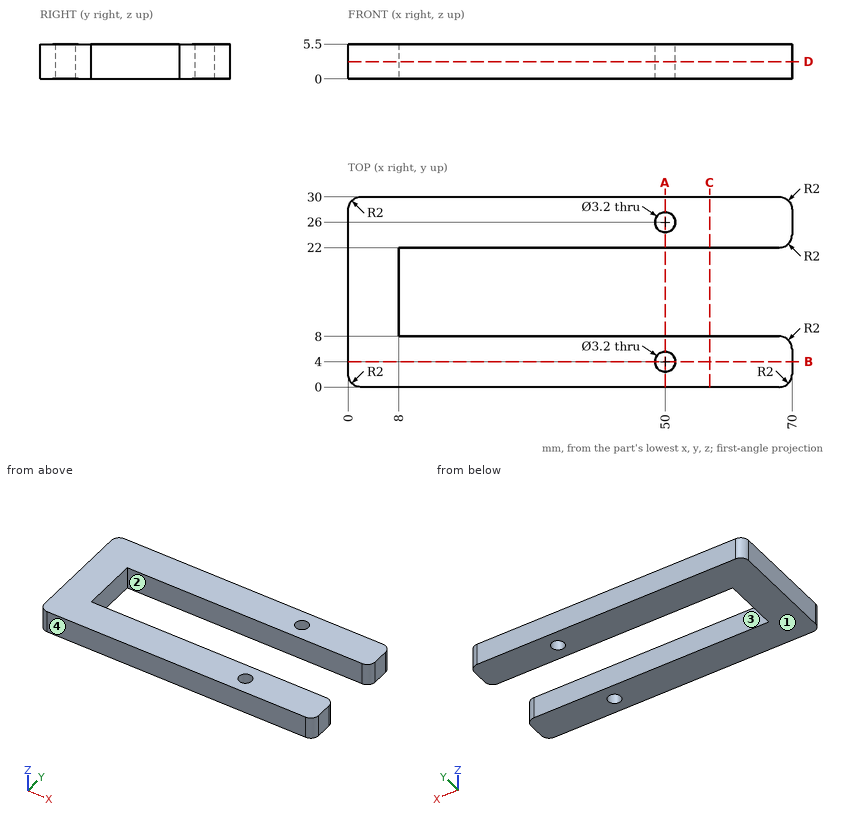
Study the drawing (mm; zero at the part's minimum x, y, z) and answer. Give positions to 0.01 mm unless a question says otherwise; leave off trailing zeros. Write each loop counter-clockwise with the first axis right and the second up, starting at its lowest first coordinate (ties: lowest second). Pieces come first, ordered by that corner, then holes.
Item 1: Section C-C, the plane x = 57 is taken. Write down the section's boundary in (y, z).
Item 2: Section D-D, the plane z = 2.7 is taken. Write down the section's boundary in (x, y), plus the area to 3 significant figures.
Item 3: Determine the mould class of the marked faces 1, 2, 3 and 4 for opening direction Y: released by +Y, released by -Y, zero draft, split by the parting line, or undercut.
Item 4: A flat-ended cylindrical pin translates along its axis: P1, Ø3, axis at y = 18.5, z = 1.5, coming from the +X side. Find the tip coordinate at first contact, or state that the pin passes through.
Item 5: Section B-B, the plane y = 4 is taken. Write down the section's boundary in (x, z).
Item 6: Find the intervals of material crossed by line 1 along Y through (x, z) = (50, 2.6); line 2 along Y through (x, z) = (18, 2.1); line 3 along X through (y, z) = (26, 2.9), in increasing order.
Item 7: Section A-A, the plane x = 50 is taken. Write down the section's boundary in (y, z), plus the area to 3 significant figures.
Completed:
1. outline: (0, 0) - (8, 0) - (8, 5.5) - (0, 5.5) - close; (22, 0) - (30, 0) - (30, 5.5) - (22, 5.5) - close
2. outline: (0, 2) arc R2 ccw to (2, 0) - (68, 0) arc R2 ccw to (70, 2) - (70, 6) arc R2 ccw to (68, 8) - (8, 8) - (8, 22) - (68, 22) arc R2 ccw to (70, 24) - (70, 28) arc R2 ccw to (68, 30) - (2, 30) arc R2 ccw to (0, 28) - close; hole circle Ø3.2 at (50, 4); hole circle Ø3.2 at (50, 26)
2. area: 1,210 mm2
3. face 1: zero draft
3. face 2: undercut
3. face 3: undercut
3. face 4: released by -Y
4. P1: stops at x = 8
5. outline: (0, 0) - (48.4, 0) - (48.4, 5.5) - (0, 5.5) - close; (51.6, 0) - (70, 0) - (70, 5.5) - (51.6, 5.5) - close
6. line 1: y = 0 to 2.4, 5.6 to 8, 22 to 24.4, 27.6 to 30
6. line 2: y = 0 to 8, 22 to 30
6. line 3: x = 0 to 48.4, 51.6 to 70
7. outline: (0, 0) - (2.4, 0) - (2.4, 5.5) - (0, 5.5) - close; (5.6, 0) - (8, 0) - (8, 5.5) - (5.6, 5.5) - close; (22, 0) - (24.4, 0) - (24.4, 5.5) - (22, 5.5) - close; (27.6, 0) - (30, 0) - (30, 5.5) - (27.6, 5.5) - close
7. area: 52.8 mm2
